Geometry: final body of the model. Coordinates: model frame, mm. A direction names the side the tool comes from. Round coordinates to 2 decimals unless told otherwise and drop trailing zeros. Order: outer loops, then holes, each group sorted by start corner. A loop starts at its lowest first (then second) coordinate and runs counter-clockwise, first axis right, second up. Notation, with made-up numbers: (-26, -8) -> (19, -8) arc R29 ccw to (19, 31) -> close; hole circle Ø5 at (30.25, 84.5). An arc over 180 degrees is marked (long way). Put each result on its own line as item: value.
```python
from build123d import *

# Parameters (mm, degrees)
SZKIC1_R                    = 1
DODANIE_WYCI_GNI_CIE1_DEPTH = 110


with BuildPart() as part:
    # Szkic1 → Dodanie-wyciągnięcie1 (new body)
    with BuildSketch(Plane.XY):
        with BuildLine():
            Line((-1.439339828, 2.5), (1.439339828, 2.5))
            Line((1.439339828, 2.5), (3.012563133, 4.073223305))
            ThreePointArc((3.012563133, 4.073223305), (3.066756321, 4.345670858), (2.835786438, 4.5))
            Line((2.835786438, 4.5), (1.25, 4.5))
            ThreePointArc((1.25, 4.5), (1.073223305, 4.573223305), (1, 4.75))
            Line((1, 4.75), (1, 5.75))
            ThreePointArc((1, 5.75), (1.073223305, 5.926776695), (1.25, 6))
            Line((1.25, 6), (5.75, 6))
            ThreePointArc((5.75, 6), (5.926776695, 5.926776695), (6, 5.75))
            Line((6, 5.75), (6, 1.25))
            ThreePointArc((6, 1.25), (5.926776695, 1.073223305), (5.75, 1))
            Line((5.75, 1), (4.75, 1))
            ThreePointArc((4.75, 1), (4.573223305, 1.073223305), (4.5, 1.25))
            Line((4.5, 1.25), (4.5, 2.835786438))
            ThreePointArc((4.5, 2.835786438), (4.345670858, 3.066756321), (4.073223305, 3.012563133))
            Line((4.073223305, 3.012563133), (2.5, 1.439339828))
            Line((2.5, 1.439339828), (2.5, -1.439339828))
            Line((2.5, -1.439339828), (4.073223305, -3.012563133))
            ThreePointArc((4.073223305, -3.012563133), (4.345670858, -3.066756321), (4.5, -2.835786438))
            Line((4.5, -2.835786438), (4.5, -1.25))
            ThreePointArc((4.5, -1.25), (4.573223305, -1.073223305), (4.75, -1))
            Line((4.75, -1), (5.75, -1))
            ThreePointArc((5.75, -1), (5.926776695, -1.073223305), (6, -1.25))
            Line((6, -1.25), (6, -5.75))
            ThreePointArc((6, -5.75), (5.926776695, -5.926776695), (5.75, -6))
            Line((5.75, -6), (1.25, -6))
            ThreePointArc((1.25, -6), (1.073223305, -5.926776695), (1, -5.75))
            Line((1, -5.75), (1, -4.75))
            ThreePointArc((1, -4.75), (1.073223305, -4.573223305), (1.25, -4.5))
            Line((1.25, -4.5), (2.835786438, -4.5))
            ThreePointArc((2.835786438, -4.5), (3.066756321, -4.345670858), (3.012563133, -4.073223305))
            Line((3.012563133, -4.073223305), (1.439339828, -2.5))
            Line((1.439339828, -2.5), (-1.439339828, -2.5))
            Line((-1.439339828, -2.5), (-3.012563133, -4.073223305))
            ThreePointArc((-3.012563133, -4.073223305), (-3.066756321, -4.345670858), (-2.835786438, -4.5))
            Line((-2.835786438, -4.5), (-1.25, -4.5))
            ThreePointArc((-1.25, -4.5), (-1.073223305, -4.573223305), (-1, -4.75))
            Line((-1, -4.75), (-1, -5.75))
            ThreePointArc((-1, -5.75), (-1.073223305, -5.926776695), (-1.25, -6))
            Line((-1.25, -6), (-5.75, -6))
            ThreePointArc((-5.75, -6), (-5.926776695, -5.926776695), (-6, -5.75))
            Line((-6, -5.75), (-6, -1.25))
            ThreePointArc((-6, -1.25), (-5.926776695, -1.073223305), (-5.75, -1))
            Line((-5.75, -1), (-4.75, -1))
            ThreePointArc((-4.75, -1), (-4.573223305, -1.073223305), (-4.5, -1.25))
            Line((-4.5, -1.25), (-4.5, -2.835786438))
            ThreePointArc((-4.5, -2.835786438), (-4.345670858, -3.066756321), (-4.073223305, -3.012563133))
            Line((-4.073223305, -3.012563133), (-2.5, -1.439339828))
            Line((-2.5, -1.439339828), (-2.5, 1.439339828))
            Line((-2.5, 1.439339828), (-4.073223305, 3.012563133))
            ThreePointArc((-4.073223305, 3.012563133), (-4.345670858, 3.066756321), (-4.5, 2.835786438))
            Line((-4.5, 2.835786438), (-4.5, 1.25))
            ThreePointArc((-4.5, 1.25), (-4.573223305, 1.073223305), (-4.75, 1))
            Line((-4.75, 1), (-5.75, 1))
            ThreePointArc((-5.75, 1), (-5.926776695, 1.073223305), (-6, 1.25))
            Line((-6, 1.25), (-6, 5.75))
            ThreePointArc((-6, 5.75), (-5.926776695, 5.926776695), (-5.75, 6))
            Line((-5.75, 6), (-1.25, 6))
            ThreePointArc((-1.25, 6), (-1.073223305, 5.926776695), (-1, 5.75))
            Line((-1, 5.75), (-1, 4.75))
            ThreePointArc((-1, 4.75), (-1.073223305, 4.573223305), (-1.25, 4.5))
            Line((-1.25, 4.5), (-2.835786438, 4.5))
            ThreePointArc((-2.835786438, 4.5), (-3.066756321, 4.345670858), (-3.012563133, 4.073223305))
            Line((-3.012563133, 4.073223305), (-1.439339828, 2.5))
        make_face()
        Circle(SZKIC1_R, mode=Mode.SUBTRACT)
    extrude(amount=-DODANIE_WYCI_GNI_CIE1_DEPTH)


solid = part.part
```
1. Cut plane A-A on y = 0. Return loops of the section in (x, z), and give its area (3 significant figures).
Ans:
outline: (-2.5, -110) -> (-1, -110) -> (-1, 0) -> (-2.5, 0) -> close; (1, -110) -> (2.5, -110) -> (2.5, 0) -> (1, 0) -> close
area: 330 mm²
2. Material intervals for probe 1 along X at (y, z) = (-1.25, -99); probe 2 along Y at (x, z) = (4.25, -55.5), sorted ascending.
Ans:
probe 1: -6 to -4.5, -2.5 to 2.5, 4.5 to 6
probe 2: -6 to -3.09, 3.09 to 6
3. Draft query along Y for faces 3 (the face through (4, -6, -54)), 4 (the face through (0.1, 1.4, 0)), 5 (the face through (-2.5, 0, -54)). Return one class per face: +Y half, -Y half, draft (parallel to the pull), parting line (faces both ways), or undercut.
Ans:
face 3: -Y half
face 4: draft
face 5: undercut
4. Contact query for a flat-ended pin moving along its axis: P1, Ø1.5, axis at y = -1, z = -91, coming from the +X side. Output: stop coordinate, or through.
Ans:
P1: x = 6
5. Set-up query: faces 1 (the face through (0, -2.5, -54)), 2 (the face through (6, 4, -54)). Return all of +Z, -Z, +X, -X, +Y, -Y with unobstructed straight access to the full face (end or side cutting, diameter ignored); none if empty.
Ans:
face 1: +Z, -Z
face 2: +Z, -Z, +X, +Y, -Y
